Can you work these out from the drawing? Everything is in mm from the part's minimum corner. A direction names the side the tool comes from. Coordinates: 2 decimals unless noted, no trailing zeros. Loops run counter-clockwise (first coordinate to the right, second up) from the corner with the lowest first, then second, coordinate; pieces in that order, holes last. Notation, with made-up numbers: (-7, 17) - (1, 17) arc R21 ccw to (1, 41) - close; hole circle Ø7 at (-4, 11.5). An arc over 180 degrees is marked (long way). Put each result on its own line as item: value. Start each with the question number.
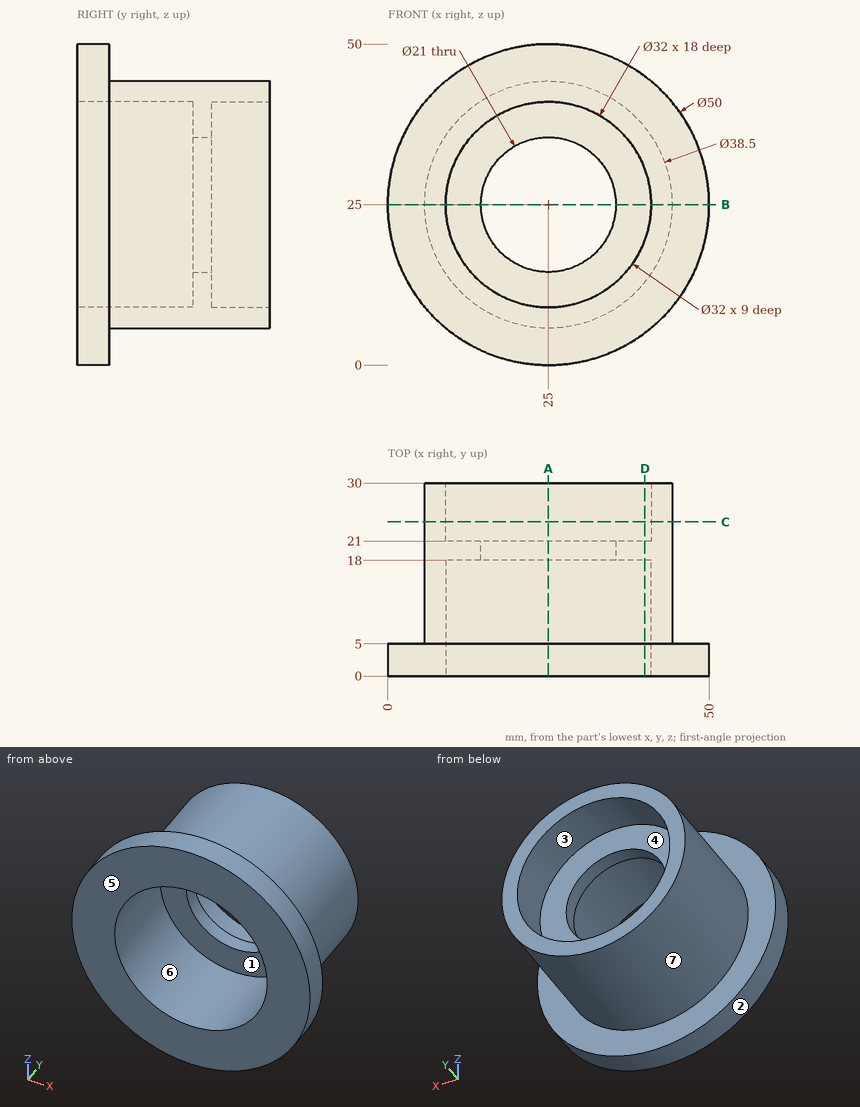
Q1. We'd pull the mould along Z, two halves only. Please class the marked faces 4, 5, 6 and 7: released by +Z, released by -Z, zero draft, split by the parting line, or undercut.
Q2. I want a section at D-D on x = 40. List the corners of the cut face in (y, z) for me.
Q3. I want a section at B-B on z = 25. List the corners of the cut face in (x, y) for me.
Q4. Will these pins go through, and if not, where does the flat tip stop? pin 1 (19 mm diameter, centred on x = 25, z = 25, fed in from +Y); pin 2 (2 mm diameter, centred on x = 8.5, y = 22.5, fed in from -Z); pin 3 (10 mm diameter, centred on x = 8, y = 18.5, fed in from -Z); pin 4 (1 mm diameter, centred on x = 36, y = 12.5, fed in from -Z).
Q5. I want a section at C-C on y = 24. List the corners of the cut face in (x, z) for me, and give its area (3 significant figures).
Q6. On a 3-axis mill with a long thin cutter (end or side, diameter ignored), from which of +Z, -Z, +X, -X, +Y, -Y can I reach the whole of each face in a straight line? I mean the marked faces 1, 2 and 3. Say none if no direction works.
Q7. I want a section at A-A on x = 25. List the corners of the cut face in (y, z) for me.
Q8. Please list where these lines run through material, in increasing order: line 1 along Z through (x, y) = (25, 19.4); line 2 along X through (y, z) = (26.25, 25); line 3 along X through (y, z) = (2, 24.5) (3 decimals). Write a range as [from, to].
Calculated:
1. face 4: undercut
1. face 5: zero draft
1. face 6: undercut
1. face 7: split by the parting line
2. outline: (0, 5) - (5, 5) - (5, 12.94) - (30, 12.94) - (30, 19.43) - (21, 19.43) - (21, 30.57) - (30, 30.57) - (30, 37.06) - (5, 37.06) - (5, 45) - (0, 45) - (0, 30.57) - (18, 30.57) - (18, 19.43) - (0, 19.43) - close
3. outline: (0, 0) - (9, 0) - (9, 18) - (14.5, 18) - (14.5, 21) - (9, 21) - (9, 30) - (5.75, 30) - (5.75, 5) - (0, 5) - close; (35.5, 18) - (41, 18) - (41, 0) - (50, 0) - (50, 5) - (44.25, 5) - (44.25, 30) - (41, 30) - (41, 21) - (35.5, 21) - close
4. pin 1: through
4. pin 2: z = 13.58
4. pin 3: z = 9.95
4. pin 4: z = 8.87
5. outline: circle Ø38.5 at (25, 25); hole circle Ø32 at (25, 25)
5. area: 360 mm2
6. face 1: -Y
6. face 2: +Y, -Y
6. face 3: +Y
7. outline: (0, 0) - (5, 0) - (5, 5.75) - (30, 5.75) - (30, 9) - (21, 9) - (21, 14.5) - (18, 14.5) - (18, 9) - (0, 9) - close; (0, 41) - (18, 41) - (18, 35.5) - (21, 35.5) - (21, 41) - (30, 41) - (30, 44.25) - (5, 44.25) - (5, 50) - (0, 50) - close
8. line 1: [5.75, 14.5], [35.5, 44.25]
8. line 2: [5.75, 9], [41, 44.25]
8. line 3: [0.005, 9.008], [40.992, 49.995]
